from build123d import *

# Parameters (mm, degrees)
SKETCH_1_R      = 1.925
EXTRUDE_1_DEPTH = 3.72
SKETCH_2_R      = 2.5
EXTRUDE_2_DEPTH = 58
EXTRUDE_START   = 4.02
SKETCH_3_R      = 1.925
EXTRUDE_3_DEPTH = 4.02


with BuildPart() as part:
    # 草图1 → 凸台-拉伸1 (new body)
    with BuildSketch(Plane.XY):
        Circle(SKETCH_1_R)
    extrude(amount=EXTRUDE_1_DEPTH)

    # 草图2 → 凸台-拉伸2 (add)
    with BuildSketch(Plane(origin=(0, 0, 0), x_dir=(-1, 0, 0), z_dir=(0, 0, -1))):
        with Locations(Location((0, 0, 0), (0, 0, 180))):
            Circle(SKETCH_2_R)
    extrude(amount=EXTRUDE_2_DEPTH)

    # 草图3 → 凸台-拉伸3 (add)
    with BuildSketch(Plane(origin=(0, 0, -58), x_dir=(-1, 0, 0), z_dir=(0, 0, -1)).offset(EXTRUDE_START)):
        with Locations(Location((0, 0, 0), (0, 0, 180))):
            Circle(SKETCH_3_R)
    extrude(amount=-EXTRUDE_3_DEPTH)


solid = part.part
The listing builds one solid part. Answer for the finished solid, in the listing's coordinates (mm). A direction names the side the tool comes from. Give positions to 0.01 mm unless a question says otherwise; leave off trailing zeros. Order: outer loops, then holes, each group sorted by start corner. A loop starts at its lowest first (then second) coordinate and runs counter-clockwise, first axis right, second up. Notation, with made-up numbers: (-8.5, 49.5) - (50.5, 49.5) arc R24 ccw to (50.5, 61.5) - close; hole circle Ø3 at (71.5, 62). An arc over 180 degrees is marked (long way). One line per item, written item: value. Start each with the question number.
1) A cutting plane is placed at A-A on y = 0. Give the vertices of the cut face in (x, z) (3 decimals).
2) Given pin 1 Ø3 at (x, z) = (-2, -48.5) entering from +Y; pin 2 Ø2 at (y, z) = (1, -49.5) entering from -X, each flat-ended and moving along its own axis, determine where each tip first touches the part or whether it passes through.
3) A cutting plane is placed at C-C on z = -2. Give the vertices of the cut face in (x, y).
4) A tool of negligible diameter and unlimited length cuts with its end or side. For faces 1 (the face through (-0.42, -1.88, 1.83)), 2 (the face through (-0.42, 1.88, -60.04)), 3 (the face through (0, 0, 3.72)), from which of +Z, -Z, +X, -X, +Y, -Y can it reach the whole face along a straight path? Write none if from no direction.
5) Find the intervals of material crossed by L1, parallel to Y at x = -0.1, z = -30; L2, parallel to Z at x = -1.5, y = 1.45; L3, parallel to X at y = 1.6, z = -46.5, in increasing order.
Answer sheet:
1. outline: (-2.5, -58) - (-1.925, -58) - (-1.925, -62.02) - (1.925, -62.02) - (1.925, -58) - (2.5, -58) - (2.5, 0) - (1.925, 0) - (1.925, 3.72) - (-1.925, 3.72) - (-1.925, 0) - (-2.5, 0) - close
2. pin 1: stops at y = 2.45
2. pin 2: stops at x = -2.5
3. outline: circle Ø5 at (0, 0)
4. face 1: +Z
4. face 2: -Z
4. face 3: +Z, +X, -X, +Y, -Y
5. L1: y = -2.5 to 2.5
5. L2: z = -58 to 0
5. L3: x = -1.92 to 1.92
